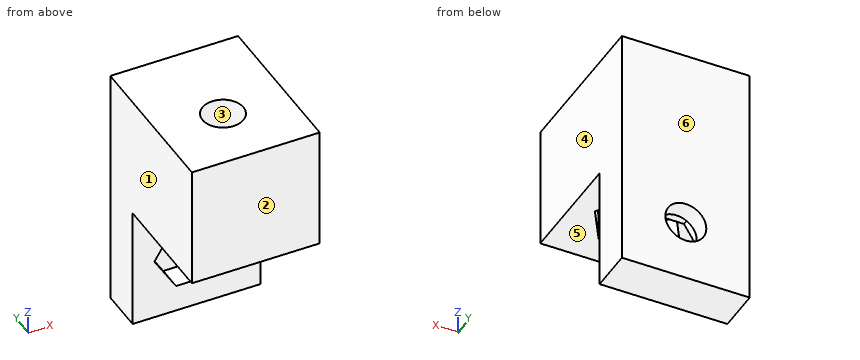
from build123d import *

# Parameters (mm, degrees)
SKETCH1_W           = 10.3
SKETCH1_H           = 12.8
SKETCH1_R           = 1.65
BOSS_EXTRUDE2_DEPTH = 5
SKETCH2_R           = 1.65
CUT_EXTRUDE1_DEPTH  = 2
SKETCH3_W           = 10.3
SKETCH3_H           = 3.5
BOSS_EXTRUDE3_DEPTH = 10
CUT_EXTRUDE2_DEPTH  = 2
SKETCH5_R           = 1.65
CUT_EXTRUDE3_DEPTH  = 1.5


with BuildPart() as part:
    # Sketch1 → Boss-Extrude2 (new, symmetric)
    with BuildSketch(Plane.XY):
        with Locations((0, 1.25)):
            Rectangle(SKETCH1_W, SKETCH1_H)
        Circle(SKETCH1_R, mode=Mode.SUBTRACT)
    extrude(amount=BOSS_EXTRUDE2_DEPTH, both=True)

    # Sketch2 → Cut-Extrude1 (cut)
    with BuildSketch(Plane(origin=(0, 0, -5), x_dir=(-1, 0, 0), z_dir=(0, 0, -1))):
        Polygon((-1.65, -2.8), (1.65, -2.8), (3.39642492, 0), (1.65, 2.8), (-1.65, 2.8), (-3.39642492, 0), align=None)
        Circle(SKETCH2_R, mode=Mode.SUBTRACT)
    extrude(amount=-CUT_EXTRUDE1_DEPTH, mode=Mode.SUBTRACT)

    # Sketch3 → Boss-Extrude3 (add)
    with BuildSketch(Plane(origin=(0, 0, -5), x_dir=(-1, 0, 0), z_dir=(0, 0, -1))):
        with Locations((0, 5.9)):
            Rectangle(SKETCH3_W, SKETCH3_H)
    extrude(amount=BOSS_EXTRUDE3_DEPTH)

    # Sketch4 → Cut-Extrude2 (cut)
    with BuildSketch(Plane.XZ.offset(-4.15)):
        with BuildLine():
            Line((-1.65, -10), (-3.39642492, -10))
            Line((-3.39642492, -10), (-1.65, -12.8))
            Line((-1.65, -12.8), (1.65, -12.8))
            Line((1.65, -12.8), (3.39642492, -10))
            Line((3.39642492, -10), (1.65, -10))
            ThreePointArc((1.65, -10), (0, -11.65), (-1.65, -10))
        make_face()
        with BuildLine():
            Line((-1.65, -7.2), (-3.39642492, -10))
            Line((-3.39642492, -10), (-1.65, -10))
            ThreePointArc((-1.65, -10), (0, -8.35), (1.65, -10))
            Line((1.65, -10), (3.39642492, -10))
            Line((3.39642492, -10), (1.65, -7.2))
            Line((1.65, -7.2), (-1.65, -7.2))
        make_face()
        with BuildLine():
            ThreePointArc((1.65, -10), (0, -8.35), (-1.65, -10))
            Line((-1.65, -10), (1.65, -10))
        make_face()
        with BuildLine():
            Line((1.65, -10), (-1.65, -10))
            ThreePointArc((-1.65, -10), (0, -11.65), (1.65, -10))
        make_face()
    extrude(amount=-CUT_EXTRUDE2_DEPTH, mode=Mode.SUBTRACT)

    # Sketch5 → Cut-Extrude3 (cut)
    with BuildSketch(Plane.XZ.offset(-6.15)):
        with Locations(Location((0, -10, 0), (0, 0, 270))):
            Circle(SKETCH5_R)
    extrude(amount=-CUT_EXTRUDE3_DEPTH, mode=Mode.SUBTRACT)


solid = part.part
The listing builds one solid part. Answer for the finished solid, in the listing's coordinates (mm). Face numbers are marked on the shaded views. A direction names the side the tool comes from. Give positions to 0.01 mm unless a question says otherwise; leave off trailing zeros. Loops run counter-clockwise (first coordinate to the right, second up) from the corner with the lowest first, then second, coordinate; pieces in that order, holes last. Notation, with made-up numbers: (3, 32.5) - (9, 32.5) arc R17 ccw to (9, 60.5) - close; hole circle Ø11 at (16.25, 83). An arc over 180 degrees is marked (long way). Write each question's results on one line, items separated by ' | '.
1. Find section C-C, the plane y = 0.5. Write down the section's boundary in (x, z).
Resolved:
outline: (-5.15, -5) - (-3.08, -5) - (-3.08, -3) - (-1.57, -3) - (-1.57, 5) - (-5.15, 5) - close; (1.57, -3) - (3.08, -3) - (3.08, -5) - (5.15, -5) - (5.15, 5) - (1.57, 5) - close
2. For a pull along X with two mould halves and no side action, classify the marked faces 1, 2, 3 and 4 as +X half, -X half, draft (parallel to the pull), parting line (faces both ways), or undercut.
Resolved:
face 1: -X half | face 2: draft | face 3: undercut | face 4: +X half
3. Find section A-A, the plane z = -3.75. Write down the section's boundary in (x, y).
Resolved:
outline: (-5.15, -5.15) - (5.15, -5.15) - (5.15, 7.65) - (-5.15, 7.65) - close; hole (-3.4, 0) - (-1.65, -2.8) - (1.65, -2.8) - (3.4, 0) - (1.65, 2.8) - (-1.65, 2.8) - close
4. Find section B-B, the plane x = 0. Write down the section's boundary in (y, z), then the cut area to 3 significant figures.
Resolved:
outline: (-5.15, -5) - (-2.8, -5) - (-2.8, -3) - (-1.65, -3) - (-1.65, 5) - (-5.15, 5) - close; (1.65, -3) - (2.8, -3) - (2.8, -5) - (4.15, -5) - (4.15, -7.2) - (6.15, -7.2) - (6.15, -8.35) - (7.65, -8.35) - (7.65, 5) - (1.65, 5) - close; (4.15, -15) - (7.65, -15) - (7.65, -11.65) - (6.15, -11.65) - (6.15, -12.8) - (4.15, -12.8) - close | area: 109 mm^2
5. Find section D-D, the plane z = -9.5. Write down the section's boundary in (x, y), then the cut area to 3 significant figures.
Resolved:
outline: (-5.15, 4.15) - (-3.08, 4.15) - (-3.08, 6.15) - (-1.57, 6.15) - (-1.57, 7.65) - (-5.15, 7.65) - close; (1.57, 6.15) - (3.08, 6.15) - (3.08, 4.15) - (5.15, 4.15) - (5.15, 7.65) - (1.57, 7.65) - close | area: 19.0 mm^2
6. Consider probe 1 along X at (y, z) = (7.3, -10); probe 2 along Y at (x, z) = (0, -1); probe 3 along Y at (x, z) = (-0.5, -4.5). Determine where each line is inside the solid, lowest interval first. Write a range as from..to.
Resolved:
probe 1: x = -5.15..-1.65, 1.65..5.15 | probe 2: y = -5.15..-1.65, 1.65..7.65 | probe 3: y = -5.15..-2.8, 2.8..7.65
7. Which of the six approach directions +Z, -Z, +X, -X, +Y, -Y give full straight-line access (tool end or side, diameter ignored) to the marked faces 5 and 6?
Resolved:
face 5: -Z, +X, -X, -Y | face 6: +Z, -Z, +X, -X, +Y
8. Flat-ended cylindrical pins translate along their axes: P1, Ø2.5, axis at x = 0, y = 0, coming from the +Z side (1 decimal); P2, Ø3, axis at x = -1.5, y = -1.5, coming from the -Z side; P3, Ø4.5, axis at x = 1, z = -9, coming from the -Y side. Find the tip coordinate at first contact, or state that the pin passes through.
Resolved:
P1: passes through | P2: stops at z = -5 | P3: stops at y = 4.15
